For this review, take the finished solid that the model builds, in its own axes (mm). Face numbers are marked on the shaded views. A direction names the side the tool comes from. Round coordinates to 2 decimals unless told otherwise and drop trailing zeros. Loops run counter-clockwise (first coordinate to the right, second up) from the corner with the lowest first, then second, coordinate; pieces in that order, holes last.
1) Mouldability with a two-part tool opening along X and no side actions: class the marked faces 1, 2, 3 and 4 as pulls with the +X half, pulls with the -X half, needs draft (parallel to the pull), parting line crosses it, or undercut.
2) Take a section at C-C (z = -0.75). State the section outline as (x, y) points.
3) Wall thickness on L1, parallel to Y at x = 0, z = -6.9; L2, parallel to Z at x = -4, y = 0.5; L3, parallel to Z at x = -0.75, y = -1: over which ranges is each line inside the solid? List them lowest first.
4) Take a section at A-A (z = -7). State the section outline as (x, y) points.
5) Insertion check: pin 1 (1.4 mm diameter, centred on x = -0.5, z = -1.5, fed in from +Y); pin 2 (1.6 mm diameter, centred on x = 0.5, y = 0, fed in from -Z); pin 3 (3 mm diameter, centred on y = 0.5, z = -1.5, fed in from +X). Each pin has a flat end and moves straight along its axis. Give the tip position at first contact, or say it passes through.
6) Tool access review of the marked faces 5, 6, 7 and 8: name each direction out of +Z, -Z, +X, -X, +Y, -Y from which nothing blocks a thin tool from reaching the whole face with its end or side.
7) Take a section at B-B (x = 0). State the section outline as (y, z) points, then the cut area to 3 significant figures.
8) Take a section at D-D (y = 2.75). State the section outline as (x, z) points, then the cut area to 3 significant figures.
```python
from build123d import *

# Parameters (mm, degrees)
PAD_DEPTH    = 3.9
PAD001_DEPTH = 6.1
SKETCH002_R  = 1.6
POCKET_DEPTH = 4.2


with BuildPart() as part:
    # Sketch → Pad (new body)
    with BuildSketch(Plane.XY):
        with BuildLine():
            Line((-3.66133, 0.49999), (-2.263681, 2.920791))
            ThreePointArc((-1.39765, 3.4208), (-1.897655, 3.286823), (-2.263681, 2.920791))
            Line((-1.39765, 3.4208), (1.39765, 3.4208))
            ThreePointArc((2.263681, 2.920791), (1.897655, 3.286823), (1.39765, 3.4208))
            Line((2.263681, 2.920791), (3.66133, 0.49999))
            ThreePointArc((3.66133, -0.49999), (3.795299, 0), (3.66133, 0.49999))
            Line((3.66133, -0.49999), (2.263681, -2.920791))
            ThreePointArc((1.39765, -3.4208), (1.897655, -3.286823), (2.263681, -2.920791))
            Line((1.39765, -3.4208), (-1.397649, -3.4208))
            ThreePointArc((-2.263681, -2.920791), (-1.897654, -3.286823), (-1.397649, -3.4208))
            Line((-2.263681, -2.920791), (-3.66133, -0.49999))
            ThreePointArc((-3.66133, 0.49999), (-3.795299, 0), (-3.66133, -0.49999))
        make_face()
    extrude(amount=PAD_DEPTH)

    # Sketch001 (on DatumPlane) → Pad001 (join)
    with BuildSketch(Plane(origin=(0, 0, 0), x_dir=(1, 0, 0), z_dir=(0, 0, -1))):
        Polygon((5, 0), (2.5, 4.330127), (-2.5, 4.330127), (-5, 0), (-2.5, -4.330127), (2.5, -4.330127), align=None)
    extrude(amount=PAD001_DEPTH)

    # Sketch002 (on DatumPlane) → Pocket (cut)
    with BuildSketch(Plane(origin=(0, 0, -6.1), x_dir=(1, 0, 0), z_dir=(0, 0, -1))):
        Circle(SKETCH002_R)
    extrude(amount=-POCKET_DEPTH, mode=Mode.SUBTRACT)


with BuildPart() as part_1:
    # Body placement: moved
    add(part.part.moved(Location((0, 0, -3.6))))


solid = part_1.part
```
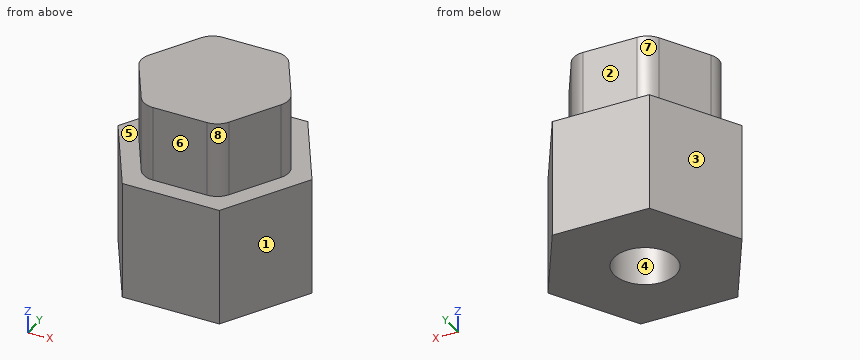
Response:
1. face 1: pulls with the +X half
1. face 2: needs draft
1. face 3: pulls with the -X half
1. face 4: undercut
2. outline: (-3.66, -0.5) - (-2.26, -2.92) arc R1 ccw to (-1.4, -3.42) - (1.4, -3.42) arc R1 ccw to (2.26, -2.92) - (3.66, -0.5) arc R1 ccw to (3.66, 0.5) - (2.26, 2.92) arc R1 ccw to (1.4, 3.42) - (-1.4, 3.42) arc R1 ccw to (-2.26, 2.92) - (-3.66, 0.5) arc R1 ccw to start
3. L1: y = -4.33 to -1.6, 1.6 to 4.33
3. L2: z = -9.7 to -3.6
3. L3: z = -5.5 to 0.3
4. outline: (-5, 0) - (-2.5, -4.33) - (2.5, -4.33) - (5, 0) - (2.5, 4.33) - (-2.5, 4.33) - close; hole circle Ø3.2 at (0, 0)
5. pin 1: stops at y = 3.42
5. pin 2: stops at z = -5.5
5. pin 3: stops at x = 3.8
6. face 5: +Z
6. face 6: +Z, +X, -X, -Y
6. face 7: +Z, -X, +Y
6. face 8: +Z, +X, -Y
7. outline: (-4.33, -9.7) - (-1.6, -9.7) - (-1.6, -5.5) - (1.6, -5.5) - (1.6, -9.7) - (4.33, -9.7) - (4.33, -3.6) - (3.42, -3.6) - (3.42, 0.3) - (-3.42, 0.3) - (-3.42, -3.6) - (-4.33, -3.6) - close
7. area: 66.1 mm2
8. outline: (-3.41, -9.7) - (3.41, -9.7) - (3.41, -3.6) - (2.36, -3.6) - (2.36, 0.3) - (-2.36, 0.3) - (-2.36, -3.6) - (-3.41, -3.6) - close
8. area: 60.1 mm2
